For this review, take the finished solid that the model builds, in its own axes (mm). Face numbers are marked on the shaded views. A direction names the side the tool comes from. Give positions to 0.01 mm unless a question says otherwise; leave off trailing zeros. Order: outer loops, then holes, each group sorted by start corner. A loop starts at its lowest first (then second) coordinate and runs counter-clockwise, first axis right, second up.
Item 1: Consider section A-A (y = 25.4). Give the boundary of the cut face in (x, z).
Item 2: The part is to be moulded in two halves that separate along Z. For the marked faces 1, 2 and 3, say which applies: released by +Z, released by -Z, zero draft, split by the parting line, or undercut.
Item 3: For P1, Ø5, axis at x = 0, y = 25.4, coming from the +Z side; P2, Ø1.5, axis at y = 21, z = 0.5, coming from the +X side; P3, Ø2, axis at x = 0.5, z = 15, coming from the -Y side, all flat-tipped, find the tip position at first contact; note any pin that passes through.
Item 4: For probe 1 along Z at (x, y) = (0, 4); probe 2 along Z at (x, y) = (0, 9.5); probe 3 along Y at (x, z) = (-2, 7), list the stretches that pass through material, from the lowest coordinate up.
Item 5: Machinability: for the marked faces 4 and 5, which of the approach directions +Z, -Z, +X, -X, +Y, -Y give a long, thin tool a straight path to every point of the face, cutting with its end or side? Answer none if there is none.
Item 6: Consider section B-B (x = 0). Give the boundary of the cut face in (y, z), plus the area to 3 significant figures.
Item 7: Consider section D-D (x = -5.25). Give the boundary of the cut face in (y, z), plus the area to 3 significant figures.
```python
from build123d import *

# Parameters (mm, degrees)
SKETCH1_W           = 41.148
SKETCH1_H           = 12.7
BOSS_EXTRUDE1_DEPTH = 9.525
SKETCH1_3_W         = 3.048
SKETCH1_3_H         = 25.4
BOSS_EXTRUDE2_DEPTH = 6.2865
SKETCH2_R           = 1.5
CUT_EXTRUDE1_DEPTH  = 23.098
SKETCH3_W           = 12.573
SKETCH3_H           = 7.85
CUT_EXTRUDE2_DEPTH  = 23.098
SKETCH4_R           = 1.5
CUT_EXTRUDE3_DEPTH  = 13.7
SKETCH5_R           = 4.7625
CUT_EXTRUDE4_DEPTH  = 6.35


with BuildPart() as part:
    # Sketch1 → Boss-Extrude1 (new body, symmetric)
    with BuildSketch(Plane(origin=(0, 0, 0), x_dir=(0, 0, -1), z_dir=(1, 0, 0))):
        with Locations((0, 6.35)):
            Rectangle(SKETCH1_W, SKETCH1_H)
    extrude(amount=BOSS_EXTRUDE1_DEPTH, both=True)

    # Sketch1_3 → Boss-Extrude2 (add, symmetric)
    with BuildSketch(Plane(origin=(0, 0, 0), x_dir=(0, 0, -1), z_dir=(1, 0, 0))):
        with Locations((0, 25.4)):
            Rectangle(SKETCH1_3_W, SKETCH1_3_H)
    extrude(amount=BOSS_EXTRUDE2_DEPTH, both=True)

    # Sketch2 → Cut-Extrude1 (cut, through all)
    with BuildSketch(Plane.XY.offset(1.524)):
        with Locations((0, 25.4)):
            Circle(SKETCH2_R)
        with Locations((0, 31.75)):
            Circle(SKETCH2_R)
    extrude(amount=-CUT_EXTRUDE1_DEPTH, mode=Mode.SUBTRACT)

    # Sketch3 → Cut-Extrude2 (cut, through all)
    with BuildSketch(Plane.XY.offset(1.524)):
        with Locations((0, 34.175)):
            Rectangle(SKETCH3_W, SKETCH3_H)
    extrude(amount=-CUT_EXTRUDE2_DEPTH, mode=Mode.SUBTRACT)

    # Sketch4 → Cut-Extrude3 (cut, through all)
    with BuildSketch(Plane(origin=(0, 12.7, 0), x_dir=(1, 0, 0), z_dir=(0, 1, 0))):
        with Locations((0, -14.224)):
            Circle(SKETCH4_R)
        with Locations((0, 14.224)):
            Circle(SKETCH4_R)
    extrude(amount=-CUT_EXTRUDE3_DEPTH, mode=Mode.SUBTRACT)

    # Sketch5 → Cut-Extrude4 (cut)
    with BuildSketch(Plane.XZ):
        with Locations((0, 14.224)):
            Circle(SKETCH5_R)
        with Locations((0, -14.224)):
            Circle(SKETCH5_R)
    extrude(amount=-CUT_EXTRUDE4_DEPTH, mode=Mode.SUBTRACT)


solid = part.part
```
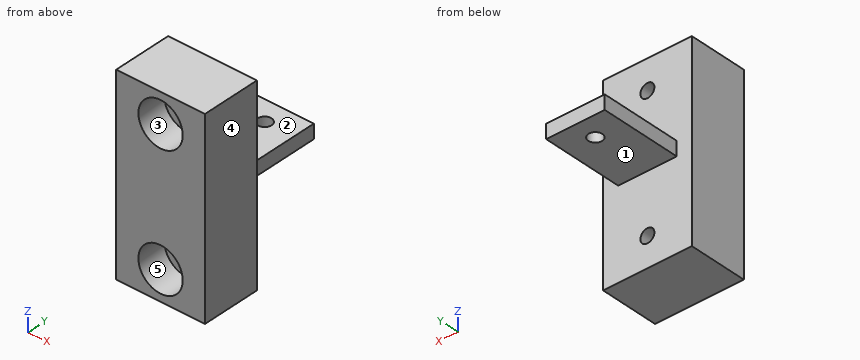
Resolved:
1. outline: (-6.29, -1.52) - (-1.5, -1.52) - (-1.5, 1.52) - (-6.29, 1.52) - close; (1.5, -1.52) - (6.29, -1.52) - (6.29, 1.52) - (1.5, 1.52) - close
2. face 1: released by -Z
2. face 2: released by +Z
2. face 3: undercut
3. P1: stops at z = 1.52
3. P2: stops at x = 6.29
3. P3: stops at y = 6.35
4. probe 1: z = -20.57 to -18.99, -9.46 to 9.46, 18.99 to 20.57
4. probe 2: z = -20.57 to -15.72, -12.72 to 12.72, 15.72 to 20.57
4. probe 3: y = 0 to 12.7
5. face 4: +Z, -Z, +X, +Y, -Y
5. face 5: -Y
6. outline: (0, -20.57) - (12.7, -20.57) - (12.7, -15.72) - (6.35, -15.72) - (6.35, -18.99) - (0, -18.99) - close; (0, -9.46) - (6.35, -9.46) - (6.35, -12.72) - (12.7, -12.72) - (12.7, -1.52) - (23.9, -1.52) - (23.9, 1.52) - (12.7, 1.52) - (12.7, 12.72) - (6.35, 12.72) - (6.35, 9.46) - (0, 9.46) - close; (0, 18.99) - (6.35, 18.99) - (6.35, 15.72) - (12.7, 15.72) - (12.7, 20.57) - (0, 20.57) - close; (26.9, -1.52) - (30.25, -1.52) - (30.25, 1.52) - (26.9, 1.52) - close
6. area: 408 mm2
7. outline: (0, -20.57) - (12.7, -20.57) - (12.7, -1.52) - (30.25, -1.52) - (30.25, 1.52) - (12.7, 1.52) - (12.7, 20.57) - (0, 20.57) - close
7. area: 576 mm2
